from build123d import *

# Parameters (mm, degrees)
SKETCH_1_R          = 6.5
EXTRUDE_1_DEPTH     = 5
SKETCH_2_W          = 12
SKETCH_2_H          = 7
SKETCH_2_W_2        = 10
SKETCH_2_H_2        = 5
EXTRUDE_1_2_DEPTH   = 5
SKETCH_3_R          = 1.2
CUT_EXTRUDE_1_DEPTH = 5
SKETCH_4_R          = 7.5
CUT_EXTRUDE_2_DEPTH = 1.1


with BuildPart() as part:
    # 草图1 → Extrude 1 (new body)
    with BuildSketch(Plane.XY):
        with BuildLine():
            Line((-10, 5), (10, 5))
            Line((10, 5), (39.072912811, 12.790063509))
            ThreePointArc((39.072912811, 12.790063509), (55.741248097, 0), (39.072912811, -12.790063509))
            Line((39.072912811, -12.790063509), (10, -5))
            Line((10, -5), (-10, -5))
            Line((-10, -5), (-39.072912811, -12.790063509))
            ThreePointArc((-39.072912811, -12.790063509), (-55.741248097, 0), (-39.072912811, 12.790063509))
            Line((-39.072912811, 12.790063509), (-10, 5))
        make_face()
        with Locations((-42.5, 0)):
            Circle(SKETCH_1_R, mode=Mode.SUBTRACT)
        with Locations((42.5, 0)):
            Circle(SKETCH_1_R, mode=Mode.SUBTRACT)
    extrude(amount=EXTRUDE_1_DEPTH)

    # 草图2 → Extrude 1 2 (add)
    with BuildSketch(Plane(origin=(0, 0, 0), x_dir=(-1, 0, 0), z_dir=(0, 0, -1))):
        Rectangle(SKETCH_2_W, SKETCH_2_H)
        Rectangle(SKETCH_2_W_2, SKETCH_2_H_2, mode=Mode.SUBTRACT)
    extrude(amount=EXTRUDE_1_2_DEPTH)

    # 草图3 → 切除-拉伸1 (cut)
    with BuildSketch(Plane(origin=(0, 0, 0), x_dir=(-1, 0, 0), z_dir=(0, 0, -1))):
        Circle(SKETCH_3_R)
    extrude(amount=-CUT_EXTRUDE_1_DEPTH, mode=Mode.SUBTRACT)

    # 草图4 → 切除-拉伸2 (cut)
    with BuildSketch(Plane(origin=(0, 0, 0), x_dir=(-1, 0, 0), z_dir=(0, 0, -1))):
        with Locations((-42.5, 0)):
            Circle(SKETCH_4_R)
        with Locations((42.5, 0)):
            Circle(SKETCH_4_R)
    extrude(amount=-CUT_EXTRUDE_2_DEPTH, mode=Mode.SUBTRACT)


solid = part.part
For this review, take the finished solid that the model builds, in its own axes (mm). A direction names the side the tool comes from. Give positions to 0.01 mm unless a question says otherwise; leave off trailing zeros. Loops run counter-clockwise (first coordinate to the right, second up) from the corner with the lowest first, then second, coordinate; pieces in that order, holes last. Notation, with made-up numbers: (20, -33) - (78, -33) arc R18 ccw to (78, -11) - close; hole circle Ø2 at (56, 37.5). An arc over 180 degrees is marked (long way). Write each question's results on one line, items separated by ' | '.
(1) For faces 4 (the flat face through (5, 0, -2)), 5 (the flat face through (-24.33, -8.84, 2.46)), 6 (the flat face through (6, 0, -2)), list the 3-axis set-ups (+Z, -Z, +X, -X, +Y, -Y) from which the entire face can be reached by the end or side of a thin tool; tool diameter is ignored.
Conclusion:
face 4: -Z | face 5: +Z, -Z, -Y | face 6: -Z, +X, +Y, -Y
(2) Take a section at A-A (x = 42.5). Give the boundary of the cut face in (y, z).
Conclusion:
outline: (-13.24, 0) - (-7.5, 0) - (-7.5, 1.1) - (-6.5, 1.1) - (-6.5, 5) - (-13.24, 5) - close; (6.5, 1.1) - (7.5, 1.1) - (7.5, 0) - (13.24, 0) - (13.24, 5) - (6.5, 5) - close
(3) For line 1 along Y through (x, z) = (-42.5, 3.5); line 2 along X through (y, z) = (-0.5, 3.5); line 3 along X through (y, z) = (1, -3.5), list the stretches that pass through material, from the lowest coordinate up.
Conclusion:
line 1: -13.24 to -6.5, 6.5 to 13.24 | line 2: -55.73 to -48.98, -36.02 to -1.09, 1.09 to 36.02, 48.98 to 55.73 | line 3: -6 to -5, 5 to 6
(4) Take a section at C-C (z = -3.25). Give the boundary of the cut face in (x, y).
Conclusion:
outline: (-6, -3.5) - (6, -3.5) - (6, 3.5) - (-6, 3.5) - close; hole (-5, -2.5) - (5, -2.5) - (5, 2.5) - (-5, 2.5) - close
(5) Take a section at D-D (y = 11.75). Give the boundary of the cut face in (x, z).
Conclusion:
outline: (-48.6, 0) - (-35.19, 0) - (-35.19, 5) - (-48.6, 5) - close; (35.19, 0) - (48.6, 0) - (48.6, 5) - (35.19, 5) - close
(6) Draft analysis for pull direction Y (two halves, no side actions). For faces 1 (the cylindrical face through (-0.65, 1.01, 2.46)), 2 (the flat face through (0, -5, 2)), 3 (the flat face through (-24.74, 8.95, 2.46)), state which applies: +Y half, -Y half, draft (parallel to the pull), parting line (faces both ways), or undercut.
Conclusion:
face 1: undercut | face 2: -Y half | face 3: +Y half
(7) For pin 1 Ø5.5 at (x, z) = (-1, -2) entering from -Y; pin 2 Ø5.5 at (x, z) = (2.5, -2) entering from +Y; pin 3 Ø4 at (y, z) = (-0.5, -3) entering from -X; pin 4 Ø10.5 at (x, y) = (42.5, 0) entering from +Z, all flat-tipped, find the tip position at first contact; note any pin that passes through.
Conclusion:
pin 1: y = -5 | pin 2: y = 5 | pin 3: x = -6 | pin 4: through
(8) Take a section at B-B (y = 0). State how many separate pieces and enclosed holes the cut face has, then the cut area to 3 significant figures.
Conclusion:
separate pieces: 4 | enclosed holes: 0 | area: 421 mm^2
